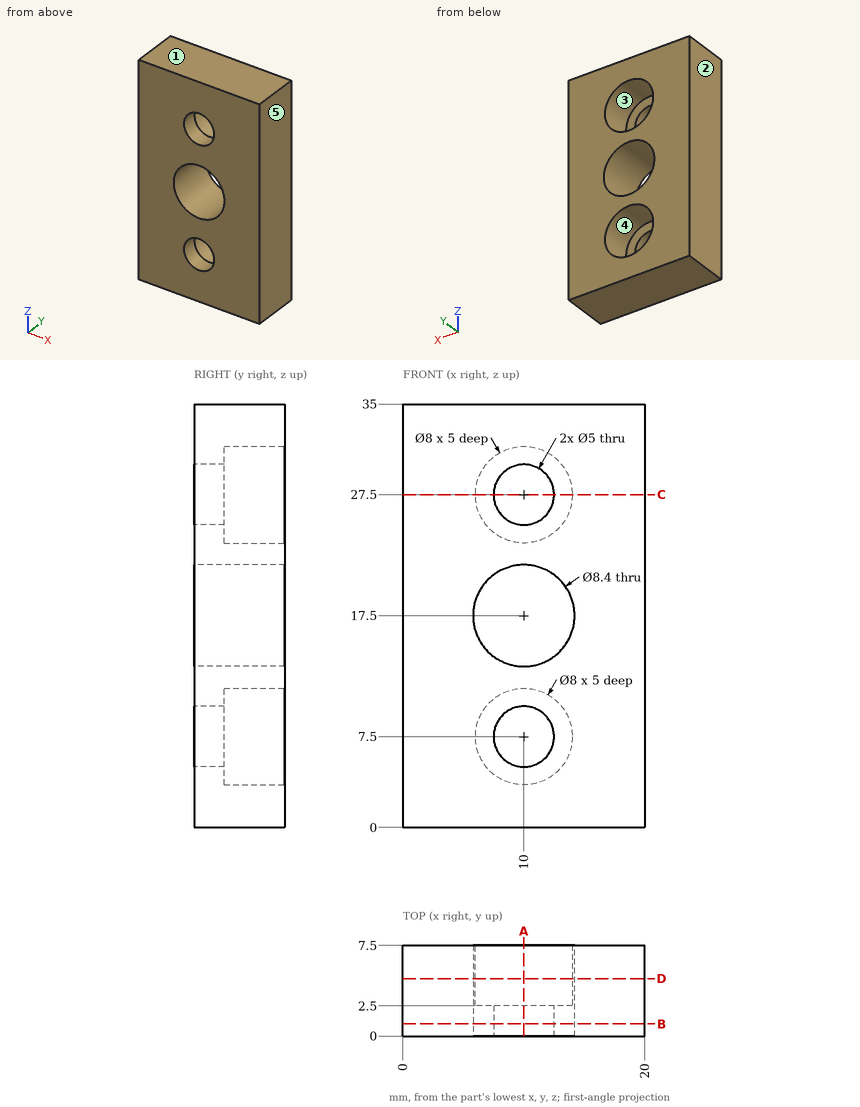
The figure shows three views and two pictorial views of one solid part (mm, origin at its lowest corner). Answer the questions. A direction names the side the tool comes from. Coordinates: 2 decimals unless noted, no trailing zeros. Loops run counter-clockwise (first coordinate to the right, second up) from the corner with the lowest first, then second, coordinate; pieces in that order, holes last. Notation, with made-up numbers: (60.25, 57) - (115.25, 57) arc R8 ccw to (115.25, 66) - close; hole circle Ø3 at (-21, 6.5). An arc over 180 degrees is marked (long way). Use a Markdown table: item, result. Add a question column.
1) The part is cut by section A-A, the plane x = 10. Give the vertices of the cut face in (y, z).
2) Find the intervals of material crossed by line 1 (Z direction, x = 10, y = 1.5); line 2 (X direction, y = 6, z = 7.5); line 3 (Z direction, x = 8, y = 5.75), in increasing order.
3) The part is cut by section B-B, the plane y = 1. Give the vertices of the cut face in (x, z), and give its area (3 significant figures).
4) For the marked faces 4 and 5, determine the directions among +Z, -Z, +X, -X, +Y, -Y from which every point of the face is accessible in a straight line to the end or side of a thin tool.
5) The part is cut by section C-C, the plane z = 27.5. Give the vertices of the cut face in (x, y), and give its area (3 significant figures).
6) The mould has two halves that part along X. Classify the marked faces 1, 2 and 3: released by +X, released by -X, zero draft, split by the parting line, or undercut.
7) The part is cut by section D-D, the plane y = 4.75. Give the vertices of the cut face in (x, z).
8) Given pin 1 (5 mm diameter, centred on x = 9, z = 18, fed in from -Y); pin 2 (2.5 mm diameter, centred on x = 8.5, z = 7.5, fed in from +Y), each flat-ended and moving along its own axis, determine where each tip first touches the part or whether it passes through.
Here are the results:
| question | item | result |
|---|---|---|
| 1 | outline | (0, 0) - (7.5, 0) - (7.5, 3.5) - (2.5, 3.5) - (2.5, 5) - (0, 5) - close; (0, 10) - (2.5, 10) - (2.5, 11.5) - (7.5, 11.5) - (7.5, 13.3) - (0, 13.3) - close; (0, 21.7) - (7.5, 21.7) - (7.5, 23.5) - (2.5, 23.5) - (2.5, 25) - (0, 25) - close; (0, 30) - (2.5, 30) - (2.5, 31.5) - (7.5, 31.5) - (7.5, 35) - (0, 35) - close |
| 2 | line 1 | z = 0 to 5, 10 to 13.3, 21.7 to 25, 30 to 35 |
| 2 | line 2 | x = 0 to 6, 14 to 20 |
| 2 | line 3 | z = 0 to 4.04, 10.96 to 13.81, 21.19 to 24.04, 30.96 to 35 |
| 3 | outline | (0, 0) - (20, 0) - (20, 35) - (0, 35) - close; hole circle Ø8.4 at (10, 17.5); hole circle Ø5 at (10, 7.5); hole circle Ø5 at (10, 27.5) |
| 3 | area | 605 mm^2 |
| 4 | face 4 | +Y |
| 4 | face 5 | +Z, -Z, +X, +Y, -Y |
| 5 | outline | (0, 0) - (7.5, 0) - (7.5, 2.5) - (6, 2.5) - (6, 7.5) - (0, 7.5) - close; (12.5, 0) - (20, 0) - (20, 7.5) - (14, 7.5) - (14, 2.5) - (12.5, 2.5) - close |
| 5 | area | 97.5 mm^2 |
| 6 | face 1 | zero draft |
| 6 | face 2 | released by -X |
| 6 | face 3 | undercut |
| 7 | outline | (0, 0) - (20, 0) - (20, 35) - (0, 35) - close; hole circle Ø8.4 at (10, 17.5); hole circle Ø8 at (10, 7.5); hole circle Ø8 at (10, 27.5) |
| 8 | pin 1 | passes through |
| 8 | pin 2 | stops at y = 2.5 |
